Source: CAD feature listing. Evaluate the final solid. Frame: model axes, mm. A direction names the side the tool comes from. Coordinates: 2 decimals unless noted, no trailing zeros. Write each loop counter-clockwise with the first axis right and the second up, starting at its lowest first coordinate (ties: lowest second). Pieces come first, ordered by that corner, then holes. Notation, with made-up numbers: (-7.75, 58) - (50.25, 58) arc R28 ccw to (50.25, 94) - close; hole circle Ø8 at (87.25, 10). An arc over 180 degrees is marked (long way). One line per item, written item: value.
from build123d import *

# Parameters (mm, degrees)
SKETCH1_W           = 139.7
SKETCH1_H           = 88.9
BOSS_EXTRUDE1_DEPTH = 63.5
SHELL1_T            = -2.54
SKETCH2_R           = 7.62
CUT_EXTRUDE1_DEPTH  = 76.2


with BuildPart() as part:
    # Sketch1 → Boss-Extrude1 (new body)
    with BuildSketch(Plane.XY):
        with Locations((11.561325185, -19.571420525)):
            Rectangle(SKETCH1_W, SKETCH1_H)
    extrude(amount=BOSS_EXTRUDE1_DEPTH)

    # Shell1
    shell1_openings = [part.faces().sort_by_distance(p)[0] for p in [
        (11.561325185, -19.571420525, 63.5),
    ]]
    offset(amount=SHELL1_T, openings=shell1_openings, kind=Kind.INTERSECTION)

    # Sketch2 → Cut-Extrude1 (cut)
    with BuildSketch(Plane(origin=(0, 0, 0), x_dir=(-1, 0, 0), z_dir=(0, 0, -1))):
        with Locations((-40.771325185, -20.31733829)):
            Circle(SKETCH2_R)
    extrude(amount=-CUT_EXTRUDE1_DEPTH, mode=Mode.SUBTRACT)


solid = part.part
1) Draft query along Y for faces 3 (the flat face through (11, -19, 2.54)), 4 (the flat face through (81.411, -20, 31)), 5 (the flat face through (11, 24.879, 31)), 6 (the flat face through (11, 22.339, 33)). Return one class per face: released by +Y, released by -Y, zero draft, split by the parting line, or undercut.
Values found:
face 3: undercut
face 4: zero draft
face 5: released by +Y
face 6: undercut
2) Section query A-A on z = 52. Output: boundary loops of the cut face in (x, y), then the cut area to 3 significant figures.
Values found:
outline: (-58.29, -64.02) - (81.41, -64.02) - (81.41, 24.88) - (-58.29, 24.88) - close; hole (-55.75, -61.48) - (78.87, -61.48) - (78.87, 22.34) - (-55.75, 22.34) - close
area: 1,140 mm2
3) Reachability of faces 1 (the flat face through (-9, -62, 63.5)), 2 (the flat face through (-55.749, -20, 33)) from +Z, -Z, +X, -X, +Y, -Y: full face, straight path, thin tool, end or side. Return the list, or none.
Values found:
face 1: +Z, +X, -X, +Y, -Y
face 2: +Z
4) Section query C-C on y = -53.5. Output: boundary loops of the cut face in (x, z).
Values found:
outline: (-58.29, 0) - (81.41, 0) - (81.41, 63.5) - (78.87, 63.5) - (78.87, 2.54) - (-55.75, 2.54) - (-55.75, 63.5) - (-58.29, 63.5) - close
5) Material intervals for line 1 (Y direction, x = -30, z = 3.5); line 2 (X direction, y = -24, z = 14); line 3 (Z direction, x = 5.5, y = -56.5), sorted ascending.
Values found:
line 1: -64.02 to -61.48, 22.34 to 24.88
line 2: -58.29 to -55.75, 78.87 to 81.41
line 3: 0 to 2.54
6) Section query B-B on x = -21. Output: boundary loops of the cut face in (y, z), then the cut area to 3 significant figures.
Values found:
outline: (-64.02, 0) - (24.88, 0) - (24.88, 63.5) - (22.34, 63.5) - (22.34, 2.54) - (-61.48, 2.54) - (-61.48, 63.5) - (-64.02, 63.5) - close
area: 535 mm2
7) Contact query for flat-ended pins moving along their axis: P1, Ø3, axis at x = -10, y = -10.5, coming from the -Z side; P2, Ø25, axis at x = 27.5, y = -39.5, coming from the +Z side. Output: stop coordinate, or through.
Values found:
P1: z = 0
P2: z = 2.54
8) Section query D-D on x = 45. Output: boundary loops of the cut face in (y, z), then the cut area to 3 significant figures.
Values found:
outline: (-64.02, 0) - (-26.66, 0) - (-26.66, 2.54) - (-61.48, 2.54) - (-61.48, 63.5) - (-64.02, 63.5) - close; (-13.98, 0) - (24.88, 0) - (24.88, 63.5) - (22.34, 63.5) - (22.34, 2.54) - (-13.98, 2.54) - close
area: 503 mm2
